Can you work these out from the model? Positions are in its coordinate system, mm. Round coordinates to 2 decimals unless told otherwise and drop trailing zeros. Write each loop counter-clockwise with the first axis right and the second up, starting at its lowest first coordinate (ties: lowest second). Pieces come first, ordered by that corner, then holes. Notation, with made-up numbers: M 82.25,-4.75 L 106.25,-4.75 A12 ccw 106.25,7.25 Z; hole C 78.5,56.5 d4. An arc over 180 degrees is marked long. Answer as a JSON object with one key per item and string values. Group by question number.
1) Please list where these lines run through material, in increasing order: L1, parallel to X at y = -37.55, z = -365.76; L2, parallel to Z at x = 16, y = -37; L3, parallel to Z at x = 16.51, y = -36.5. Write a range as [from, to].
2) If we mould it in two halves opening along Z, with no side actions, what happens to faces 1 (the flat face through (249, -38.1, -6)), 2 (the flat face through (351, -35.56, -179)), 3 (the flat face through (350.64, -13.8, -354.16))? For each: +Z half, -Z half, draft (parallel to the pull), parting line (faces both ways), or undercut.
3) Suppose I cut it at A-A, the plane x = 612. Write out the boundary of the cut face in (y, z).
4) I'm going to push flat-ended pins straight in: pin 1 Ø2 at (x, y) = (25, -37) entering from -Z; pin 2 Ø12 at (y, z) = (-13, -223) entering from +X; pin 3 Ø8 at (x, z) = (456.5, -138) entering from -Y. Where does each tip first touch, or does it pass through?
5) Suppose I cut it at B-B, the plane z = -232. Write out the boundary of the cut face in (x, y).
6) Suppose I cut it at C-C, the plane y = -15. Write out the boundary of the cut face in (x, z).
from build123d import *

# Parameters (mm, degrees)
F0_W     = 711.2
F0_H     = 368.3
F1_DEPTH = 38.1
F2_W     = 685.8
F2_H     = 336.55
F3_DEPTH = 2.54
F4_W     = 5.08
F4_H     = 5.08
F4_R     = 1.651
F5_DEPTH = 2.54
F6_DEPTH = 2.54
F7_SIZE  = 27.94
F8_R     = 5.08


with BuildPart() as f1:
    # F0 (on Front) → F1 (new body)
    with BuildSketch(Plane.XZ):
        with Locations((355.6, -184.15)):
            Rectangle(F0_W, F0_H)
    extrude(amount=F1_DEPTH)

    # F2 (on face) → F3 (cut)
    with BuildSketch(Plane.XZ.offset(38.1)):
        with Locations((355.6, -180.975)):
            Rectangle(F2_W, F2_H)
    extrude(amount=-F3_DEPTH, mode=Mode.SUBTRACT)

    # F4 (on face) → F5 (cut)
    with BuildSketch(Plane.XZ.offset(38.1)):
        with Locations((24.13, -365.76)):
            Rectangle(F4_W, F4_H)
        with Locations((43.18, -365.76)):
            Rectangle(F4_W, F4_H)
        with Locations((36.83, -365.76)):
            Rectangle(F4_W, F4_H)
        with Locations((30.48, -365.76)):
            Rectangle(F4_W, F4_H)
        with Locations((16.51, -365.76)):
            Circle(F4_R)
    extrude(amount=-F5_DEPTH, mode=Mode.SUBTRACT)

    # F4 (on face) → F6 (cut)
    with BuildSketch(Plane.XZ.offset(38.1)):
        with Locations((24.13, -365.76)):
            Rectangle(F4_W, F4_H)
        with Locations((43.18, -365.76)):
            Rectangle(F4_W, F4_H)
        with Locations((36.83, -365.76)):
            Rectangle(F4_W, F4_H)
        with Locations((30.48, -365.76)):
            Rectangle(F4_W, F4_H)
        with Locations((16.51, -365.76)):
            Circle(F4_R)
    extrude(amount=-F6_DEPTH, mode=Mode.SUBTRACT)

    # F7
    f7_edges = [f1.edges().sort_by_distance(p)[0] for p in [
        (355.6, 0, -368.3),
        (0, 0, -184.15),
        (711.2, 0, -184.15),
        (355.6, 0, 0),
    ]]
    chamfer(f7_edges, length=F7_SIZE)

    # F8
    f8_edges = [f1.edges().sort_by_distance(p)[0] for p in [
        (683.26, 0, -184.15),
        (355.6, 0, -340.36),
        (27.94, 0, -184.15),
        (355.6, 0, -27.94),
        (711.2, -27.94, -184.15),
        (355.6, -27.94, 0),
        (355.6, -27.94, -368.3),
        (0, -27.94, -184.15),
    ]]
    fillet(f8_edges, radius=F8_R)


solid = f1.part
Results:
{
 "1": {"L1": "[0, 14.86], [18.16, 21.59], [26.67, 27.94], [33.02, 34.29], [39.37, 40.64], [45.72, 711.2]", "L2": "[-368.3, -367.33], [-364.19, -349.25], [-12.7, 0]", "L3": "[-368.3, -367.41], [-364.11, -349.25], [-12.7, 0]"},
 "2": {"face 1": "draft", "face 2": "undercut", "face 3": "-Z half"},
 "3": {"outline": "M -38.1,-368.3 L -30.04,-368.3 A5.08 ccw -26.45,-366.81 L -1.49,-341.85 A5.08 ccw 0,-338.26 L 0,-30.04 A5.08 ccw -1.49,-26.45 L -26.45,-1.49 A5.08 ccw -30.04,0 L -38.1,0 L -38.1,-12.7 L -35.56,-12.7 L -35.56,-349.25 L -38.1,-349.25 Z"},
 "4": {"pin 1": "z = -363.22", "pin 2": "x = 702.26", "pin 3": "y = -35.56"},
 "5": {"outline": "M 0,-38.1 L 12.7,-38.1 L 12.7,-35.56 L 698.5,-35.56 L 698.5,-38.1 L 711.2,-38.1 L 711.2,-30.04 A5.08 ccw 709.71,-26.45 L 684.75,-1.49 A5.08 ccw 681.16,0 L 30.04,0 A5.08 ccw 26.45,-1.49 L 1.49,-26.45 A5.08 ccw 0,-30.04 Z"},
 "6": {"outline": "M 12.94,-355.36 L 698.26,-355.36 L 698.26,-12.94 L 12.94,-12.94 Z"}
}
